Design review of the part shown in the three views and the two pictorial views. Dimensions are in mm from the part's minimum x, y and z. A direction names the side the tool comes from. Give positions to 0.01 mm unless a question says otherwise; leave off trailing zeros. Order: outer loops, then holes, each group sorted by start corner. A loop starts at its lowest first (then second) coordinate and runs counter-clockwise, first axis right, second up.
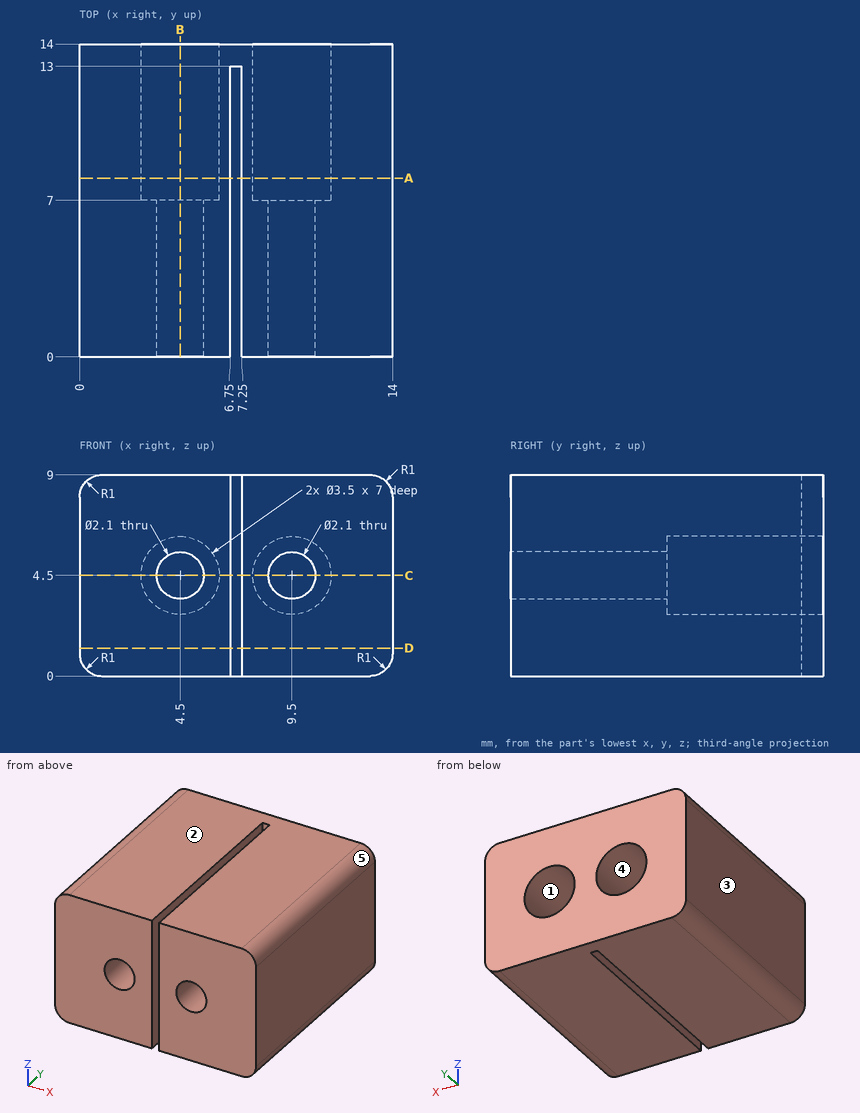
1) We need section C-C on z = 4.5. Give the boundary of the cut face in (x, y).
Answer sheet:
outline: (0, 0) - (3.45, 0) - (3.45, 7) - (2.75, 7) - (2.75, 14) - (0, 14) - close; (5.55, 0) - (6.75, 0) - (6.75, 13) - (7.25, 13) - (7.25, 0) - (8.45, 0) - (8.45, 7) - (7.75, 7) - (7.75, 14) - (6.25, 14) - (6.25, 7) - (5.55, 7) - close; (10.55, 0) - (14, 0) - (14, 14) - (11.25, 14) - (11.25, 7) - (10.55, 7) - close
2) We need section D-D on z = 1.25. Give the boundary of the cut face in (x, y).
Answer sheet:
outline: (0, 0) - (6.75, 0) - (6.75, 13) - (7.25, 13) - (7.25, 0) - (14, 0) - (14, 14) - (0, 14) - close
3) Tool access review of the marked faces 4 and 5: name each direction out of +Z, -Z, +X, -X, +Y, -Y from which nothing blocks a thin tool from reaching the whole face with its end or side.
Answer sheet:
face 4: +Y
face 5: +Z, +X, +Y, -Y
4) Draft analysis for pull direction X (two halves, no side actions). For the marked faces 1, 2 and 3, state which applies: +X half, -X half, draft (parallel to the pull), parting line (faces both ways), or undercut.
Answer sheet:
face 1: undercut
face 2: draft
face 3: -X half
5) To check wall thickness, follow line 1 (X direction, y = 9.5, z = 4.5); line 2 (X direction, y = 3, z = 4.5); line 3 (Z direction, x = 9.5, y = 12.5). State the ranges of each line that lie inside material, in increasing order.
Answer sheet:
line 1: x = 0 to 2.75, 6.25 to 6.75, 7.25 to 7.75, 11.25 to 14
line 2: x = 0 to 3.45, 5.55 to 6.75, 7.25 to 8.45, 10.55 to 14
line 3: z = 0 to 2.75, 6.25 to 9
6) We need section A-A on y = 8. Give the boundary of the cut face in (x, z), then the cut area to 3 significant figures.
Answer sheet:
outline: (0, 1) arc R1 ccw to (1, 0) - (6.75, 0) - (6.75, 9) - (1, 9) arc R1 ccw to (0, 8) - close; (7.25, 0) - (13, 0) arc R1 ccw to (14, 1) - (14, 8) arc R1 ccw to (13, 9) - (7.25, 9) - close; hole circle Ø3.5 at (4.5, 4.5); hole circle Ø3.5 at (9.5, 4.5)
area: 101 mm2
7) Clearance check with a flat-ended pin moving along its axis: pin 1 (1.8 mm diameter, centred on x = 9.5, z = 4.5, fed in from +Y) (3 decimals). State where the tip first meets the part, or that it passes through.
Answer sheet:
pin 1: passes through
8) We need section B-B on x = 4.5. Give the boundary of the cut face in (y, z).
Answer sheet:
outline: (0, 0) - (14, 0) - (14, 2.75) - (7, 2.75) - (7, 3.45) - (0, 3.45) - close; (0, 5.55) - (7, 5.55) - (7, 6.25) - (14, 6.25) - (14, 9) - (0, 9) - close
